For this review, take the finished solid that the model builds, in its own axes (mm). A direction names the side the tool comes from. Coordinates: 2 decimals unless noted, no trailing zeros. Loops run counter-clockwise (first coordinate to the right, second up) from the corner with the lowest first, then second, coordinate; pieces in that order, holes last. Notation, with made-up numbers: (85.5, 89.25) -> (121.5, 89.25) arc R18 cw to (121.5, 123.25) -> close; hole circle Ø6 at (22.25, 68). An arc over 180 degrees is marked (long way). Answer in a Markdown table with one row per item.
from build123d import *

# Parameters (mm, degrees)
SKETCH1_R           = 7
BOSS_EXTRUDE1_DEPTH = 4.7625
FILLET1_R           = 2.5
CHAMFER1_SIZE       = 1
SKETCH3_R           = 7
SKETCH3_R_2         = 6
BOSS_EXTRUDE2_DEPTH = 2


with BuildPart() as part:
    # Sketch1 → Boss-Extrude1 (new, symmetric)
    with BuildSketch(Plane(origin=(0, 0, 0), x_dir=(1, 0, 0), z_dir=(0, 1, 0))):
        with BuildLine():
            Line((-30.675, 0), (-30.675, 6.35))
            Line((-30.675, 6.35), (-5, 6.35))
            Line((-5, 6.35), (-5, 28.341685226))
            ThreePointArc((-5, 28.341685226), (0, 44.825), (5, 28.341685226))
            Line((5, 28.341685226), (5, 6.35))
            Line((5, 6.35), (30.675, 6.35))
            Line((30.675, 6.35), (30.675, 0))
            Line((30.675, 0), (-30.675, 0))
        make_face()
        with Locations(Location((0, 35.825, 0), (0, 0, 90))):
            Circle(SKETCH1_R, mode=Mode.SUBTRACT)
    extrude(amount=BOSS_EXTRUDE1_DEPTH, both=True)

    # Fillet1
    fillet1_edges = [part.edges().sort_by_distance(p)[0] for p in [
        (-30.675, 0, -6.35),
        (-5, 0, -6.35),
        (-5, 0, -28.341685226),
        (5, 0, -28.341685226),
        (5, 0, -6.35),
        (30.675, 0, -6.35),
    ]]
    fillet(fillet1_edges, radius=FILLET1_R)

    # Chamfer1
    chamfer1_edges = [part.edges().sort_by_distance(p)[0] for p in [
        (30.675, -4.7625, -1.925),
        (-5, -4.7625, -17.978601056),
        (-5, 4.7625, -17.978601056),
        (0, -4.7625, -44.825),
        (0, 4.7625, -44.825),
        (5, -4.7625, -17.978601056),
        (5, 4.7625, -17.978601056),
        (17.8375, -4.7625, -6.35),
        (17.8375, 4.7625, -6.35),
        (-30.675, -4.7625, -1.925),
        (-17.8375, -4.7625, -6.35),
        (-29.942766953, -4.7625, -5.617766953),
        (29.942766953, -4.7625, -5.617766953),
        (-17.8375, 4.7625, -6.35),
        (-30.675, 4.7625, -1.925),
        (-29.942766953, 4.7625, -5.617766953),
        (29.942766953, 4.7625, -5.617766953),
        (-5.227766852, -4.7625, -28.149774183),
        (-5.227766852, 4.7625, -28.149774183),
        (5.227766852, -4.7625, -28.149774183),
        (5.227766852, 4.7625, -28.149774183),
        (5.732233047, -4.7625, -7.082233047),
        (5.732233047, 4.7625, -7.082233047),
        (-5.732233047, -4.7625, -7.082233047),
        (-5.732233047, 4.7625, -7.082233047),
        (30.675, 4.7625, -1.925),
    ]]
    chamfer(chamfer1_edges, length=CHAMFER1_SIZE)

    # Sketch3 → Boss-Extrude2 (add, symmetric)
    with BuildSketch(Plane(origin=(0, 0, 0), x_dir=(1, 0, 0), z_dir=(0, 1, 0))):
        with Locations(Location((0, 35.825, 0), (0, 0, 90))):
            Circle(SKETCH3_R)
        with Locations(Location((0, 35.825, 0), (0, 0, 270))):
            Circle(SKETCH3_R_2, mode=Mode.SUBTRACT)
    extrude(amount=BOSS_EXTRUDE2_DEPTH, both=True)


solid = part.part
Item 1: Take a section at B-B, the plane y = 0. State the section outline as (x, z) points (3 decimals), and give its area (3 significant figures).
Worked answers:
| item | result |
|---|---|
| outline | (-30.675, -3.85) arc R2.5 ccw to (-28.175, -6.35) -> (-7.5, -6.35) arc R2.5 cw to (-5, -8.85) -> (-5, -27.107) arc R2.5 cw to (-5.87, -29.002) arc R9 ccw (long way) to (5.87, -29.002) arc R2.5 cw to (5, -27.107) -> (5, -8.85) arc R2.5 cw to (7.5, -6.35) -> (28.175, -6.35) arc R2.5 ccw to (30.675, -3.85) -> (30.675, 0) -> (-30.675, 0) -> close; hole circle Ø12 at (0, -35.825) |
| area | 741 mm² |
Item 2: Take a section at C-C, the plane x = 20. State the section outline as (y, z) points, and give its area (3 significant figures).
Worked answers:
| item | result |
|---|---|
| outline | (-4.76, -5.35) -> (-3.76, -6.35) -> (3.76, -6.35) -> (4.76, -5.35) -> (4.76, 0) -> (-4.76, 0) -> close |
| area | 59.5 mm² |
Item 3: Insertion check: pin 1 (1 mm diameter, centred on x = 10, y = -0.5, fed in from -Z); pin 2 (2.5 mm diameter, centred on y = -1, z = -14.5, fed in from +X); pin 3 (3 mm diameter, centred on x = 6, y = 3.5, fed in from -Z). Each pin has a flat end and moves straight along its axis. Give the tip position at first contact, or say it passes through.
Worked answers:
| item | result |
|---|---|
| pin 1 | z = -6.35 |
| pin 2 | x = 5 |
| pin 3 | z = -43.62 |
Item 4: Take a section at D-D, the plane z = -18.5. State the section outline as (x, y) points.
Worked answers:
| item | result |
|---|---|
| outline | (-5, -3.76) -> (-4, -4.76) -> (4, -4.76) -> (5, -3.76) -> (5, 3.76) -> (4, 4.76) -> (-4, 4.76) -> (-5, 3.76) -> close |
Item 5: Take a section at A-A, the plane x = 0. State the section outline as (y, z) points (1 decimal).
Worked answers:
| item | result |
|---|---|
| outline | (-4.8, -43.8) -> (-3.8, -44.8) -> (3.8, -44.8) -> (4.8, -43.8) -> (4.8, -42.8) -> (2, -42.8) -> (2, -41.8) -> (-2, -41.8) -> (-2, -42.8) -> (-4.8, -42.8) -> close; (-4.8, -28.8) -> (-2, -28.8) -> (-2, -29.8) -> (2, -29.8) -> (2, -28.8) -> (4.8, -28.8) -> (4.8, 0) -> (-4.8, 0) -> close |
Item 6: For L1, parallel to X at y = 2.25, z = -35.5; L2, parallel to Z at x = -11, y = -1.5; L3, parallel to X at y = -2.25, z = -16.5, list the stretches that pass through material, from the lowest coordinate up.
Worked answers:
| item | result |
|---|---|
| L1 | -8.99 to -6.99, 6.99 to 8.99 |
| L2 | -6.35 to 0 |
| L3 | -5 to 5 |
Item 7: The part is to be moulded in two halves that separate along Z. For faces 1 (the flat face through (0, -4.762, -9)), 2 (the cylindrical face through (5.713, 0.053, -7.102)), 3 (the flat face through (0, 0, 0)), say which applies: +Z half, -Z half, draft (parallel to the pull), parting line (faces both ways), or undercut.
Worked answers:
| item | result |
|---|---|
| face 1 | draft |
| face 2 | undercut |
| face 3 | +Z half |
Item 8: For faces 4 (the cylindrical face through (-0.31, -3.4, -28.83)), 5 (the flat face through (5, 0, -18)), 6 (the flat face through (6, 2, -38)), 7 (the conical face through (-5.485, 4.144, -6.79)), list the 3-axis set-ups (+Z, -Z, +X, -X, +Y, -Y) from which the entire face can be reached by the end or side of a thin tool; tool diameter is ignored.
Worked answers:
| item | result |
|---|---|
| face 4 | -Y |
| face 5 | +X, +Y, -Y |
| face 6 | +Y |
| face 7 | -X, +Y |
